Study the drawing (mm; zero at the part's minimum x, y, z) and answer. A direction names the side the tool comes from. Round coordinates to 2 decimals unless told otherwise and drop trailing zeros. Write each loop counter-clockwise with the first axis right and the second up, starting at its lowest first coordinate (ties: lowest second). Pieces come first, ordered by that corner, then holes. Notation, with made-up numbers: (66, 50.5) - (103, 50.5) arc R22 cw to (103, 79.5) - close; hole circle Ø9 at (70, 61.5). An arc over 180 degrees is marked (long way). Use one line per item in the form item = value. Start each with the question number.
1) For a pull along X with two mould halves and no side action, classify the marked faces 3, 4 and 5 as released by +X, released by -X, zero draft, split by the parting line, or undercut.
2) The part is cut by section A-A, the plane z = 24. Give the vertices of the cut face in (x, y).
3) Consider line 1 along X through (y, z) = (23, 21); line 2 along X through (y, z) = (7.5, 37.5) (1 decimal); line 3 along X through (y, z) = (31.5, 43.5). Determine where each line is inside the solid, lowest interval first. Write a range as from..to.
4) The part is cut by section D-D, the plane x = 28. Give the vertices of the cut face in (y, z) (1 decimal).
5) Each of these flat-tipped pins is pushed along its axis until it touches: pin 1 (4 mm diameter, centred on x = 6.5, z = 6, fed in from +Y); pin 2 (4 mm diameter, centred on y = 15.79, z = 16.81, fed in from +X). Where does it stop, or does it pass through?
6) For the marked faces 1 and 2, determine the directions among +Z, -Z, +X, -X, +Y, -Y from which every point of the face is accessible in a straight line to the end or side of a thin tool.
7) The part is cut by section B-B, the plane y = 5. Give the vertices of the cut face in (x, z), plus the area to 3 significant figures.
8) The part is cut by section C-C, the plane z = 18. Give the vertices of the cut face in (x, y) (1 decimal), plus the area to 3 significant figures.
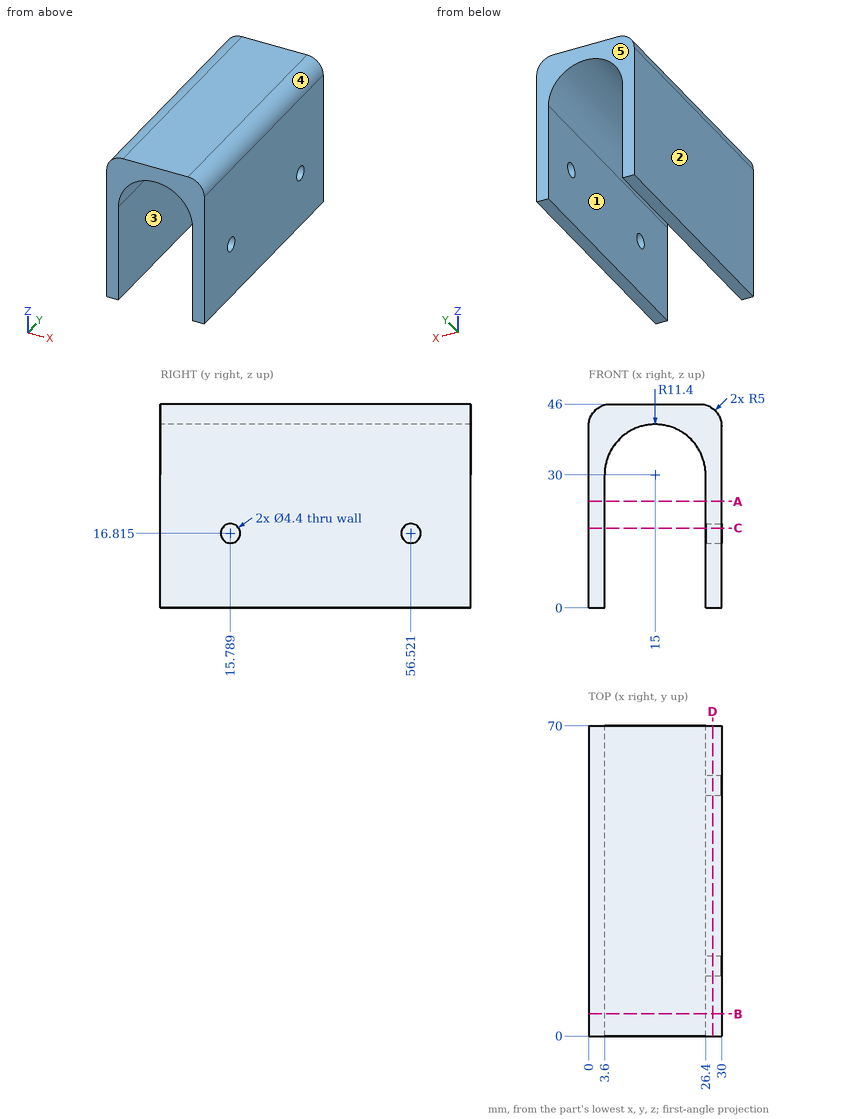
Geometry results:
q1.face_3 = undercut
q1.face_4 = released by +X
q1.face_5 = zero draft
q2.outline = (0, 0) - (3.6, 0) - (3.6, 70) - (0, 70) - close; (26.4, 0) - (30, 0) - (30, 70) - (26.4, 70) - close
q3.line_1 = 0..3.6, 26.4..30
q3.line_2 = 0..6.4, 23.6..30
q3.line_3 = 0.67..29.33
q4.outline = (0, 0) - (70, 0) - (70, 45) - (0, 45) - close; hole circle Ø4.4 at (15.8, 16.8); hole circle Ø4.4 at (56.5, 16.8)
q5.pin_1 = through
q5.pin_2 = 3.6
q6.face_1 = -Z, +Y, -Y
q6.face_2 = +Z, -Z, -X, +Y, -Y
q7.outline = (0, 0) - (3.6, 0) - (3.6, 30) arc R11.4 cw to (26.4, 30) - (26.4, 0) - (30, 0) - (30, 41) arc R5 ccw to (25, 46) - (5, 46) arc R5 ccw to (0, 41) - close
q7.area = 481 mm2
q8.outline = (0, 0) - (3.6, 0) - (3.6, 70) - (0, 70) - close; (26.4, 0) - (30, 0) - (30, 13.9) - (26.4, 13.9) - close; (26.4, 17.6) - (30, 17.6) - (30, 54.7) - (26.4, 54.7) - close; (26.4, 58.4) - (30, 58.4) - (30, 70) - (26.4, 70) - close
q8.area = 477 mm2
